```python
from build123d import *

# Parameters (mm, degrees)
SKETCH1_R           = 17.145
SKETCH1_R_2         = 1.436229084
BOSS_EXTRUDE1_DEPTH = 2.38125
SKETCH3_R           = 2.794
BOSS_EXTRUDE2_DEPTH = 3.175
BOSS_EXTRUDE3_DEPTH = 1.524
SKETCH5_W           = 5.08
SKETCH5_H           = 3.81
SKETCH5_W_2         = 3.81
SKETCH5_H_2         = 5.08
BOSS_EXTRUDE4_DEPTH = 2.159


with BuildPart() as part:
    # Sketch1 → Boss-Extrude1 (new body)
    with BuildSketch(Plane(origin=(0, 0, 0), x_dir=(1, 0, 0), z_dir=(0, 1, 0))):
        with Locations(Location((-9.270876778, 8.817912865, 0), (0, 0, 90))):
            Circle(SKETCH1_R)
        with Locations(Location((-9.270876778, 8.817912865, 0), (0, 0, 90))):
            Circle(SKETCH1_R_2, mode=Mode.SUBTRACT)
    extrude(amount=BOSS_EXTRUDE1_DEPTH)

    # Sketch3 → Boss-Extrude2 (add)
    with BuildSketch(Plane(origin=(0, 2.38125, 0), x_dir=(1, 0, 0), z_dir=(0, 1, 0))):
        with Locations(Location((-16.007627964, 14.618626912, 0), (0, 0, 270))):
            Circle(SKETCH3_R)
    extrude(amount=BOSS_EXTRUDE2_DEPTH)

    # Sketch4 → Boss-Extrude3 (add)
    with BuildSketch(Plane(origin=(0, 2.38125, 0), x_dir=(1, 0, 0), z_dir=(0, 1, 0))):
        Polygon((-10.391608677, -0.001160783), (-3.867194412, 6.037391899), (-1.106713185, 3.054802521), (-7.63112745, -2.983750162), (-10.046548523, -0.373984456), align=None)
    extrude(amount=BOSS_EXTRUDE3_DEPTH)

    # Sketch5 → Boss-Extrude4 (add)
    with BuildSketch(Plane(origin=(0, 2.38125, 0), x_dir=(1, 0, 0), z_dir=(0, 1, 0))):
        with Locations((-9.905876778, -5.787087135)):
            Rectangle(SKETCH5_W, SKETCH5_H)
        with Locations((-9.062799481, 23.422912865)):
            Rectangle(SKETCH5_W, SKETCH5_H)
        with Locations((-23.875876778, 9.452912865)):
            Rectangle(SKETCH5_W_2, SKETCH5_H_2)
        with Locations((5.334123222, 9.452912865)):
            Rectangle(SKETCH5_W_2, SKETCH5_H_2)
    extrude(amount=BOSS_EXTRUDE4_DEPTH)


solid = part.part
```
Could you check a few things on this model? Use its own coordinates, in mm. A direction names the side the tool comes from. Give positions to 0.01 mm unless a question says otherwise; leave off trailing zeros. Order: outer loops, then holes, each group sorted by start corner. A loop starts at its lowest first (then second) coordinate and runs counter-clockwise, first axis right, second up.
Q1. Suppose I cut it at B-B, the plane x = -3. Write out the boundary of the cut face in (y, z).
Q2. Suppose I cut it at C-C, the plane y = 0.65. Write out the boundary of the cut face in (x, z) (3 decimals).
Q3. If I drill on line 1 along X through (y, z) = (2.75, -7.5); line 2 along Z through (x, y) = (-10.5, 3.85); line 3 along Y through (x, z) = (-10.5, 3), over which ranges is the centre line in solid material (lowest first)?
Q4. I'm going to push flat-ended pins straight in: P1, Ø12, axis at x = -9.5, z = -5, coming from the +Y side; P2, Ø4, axis at x = -5.5, z = -9, coming from the +Y side; P3, Ø0.6, axis at y = 4, z = -10.5, coming from the +X side. Where does each tip first touch, or does it pass through?
Q5. Suppose I cut it at A-A, the plane z = -12.5. Write out the boundary of the cut face in (x, y).
Q6. Suppose I cut it at D-D, the plane x = 1. Write out the boundary of the cut face in (y, z), and give its area (3 significant figures).
Q7. For faces 5 (the flat face through (-6.523, 3, -23)), 6 (the flat face through (-24, 3, -6.913)), 7 (the flat face through (-24, 3, -11.993)), 8 (the flat face through (-25.781, 3, -9)), which set-ups out of +Z, -Z, +X, -X, +Y, -Y let a thin tool reach every point of the face, with its end or its side?
Q8. We'd pull the mould along Z, two halves only. Please class faces 1 (the flat face through (-7.175, 3.133, -2.976)), 2 (the flat face through (-11.603, 3, -23)), 3 (the flat face through (-10, 3, 3.882)), 4 (the cylindrical face through (-17.08, 3.95, -12.04)): +Z half, -Z half, draft (parallel to the pull), parting line (faces both ways), or undercut.
Solution:
1. outline: (0, -24.77) - (2.38, -24.77) - (2.38, -5.1) - (3.91, -5.1) - (3.91, -1.3) - (2.38, -1.3) - (2.38, 7.14) - (0, 7.14) - close
2. outline: circle Ø34.29 at (-9.271, -8.818); hole circle Ø2.872 at (-9.271, -8.818)
3. line 1: x = -25.78 to -21.97, 3.43 to 7.24
3. line 2: z = -25.33 to -21.52, 3.88 to 7.69
3. line 3: y = 0 to 2.38
4. P1: stops at y = 3.91
4. P2: stops at y = 2.38
4. P3: stops at x = 7.24
5. outline: (-26.02, 0) - (7.47, 0) - (7.47, 2.38) - (-14.19, 2.38) - (-14.19, 5.56) - (-17.83, 5.56) - (-17.83, 2.38) - (-26.02, 2.38) - close
6. outline: (0, -22.55) - (2.38, -22.55) - (2.38, 4.91) - (0, 4.91) - close
6. area: 65.4 mm2
7. face 5: -Z, +X, +Y
7. face 6: +Z, +X, -X, +Y
7. face 7: -Z, -X, +Y
7. face 8: +Z, -Z, -X, +Y
8. face 1: undercut
8. face 2: draft
8. face 3: undercut
8. face 4: parting line
